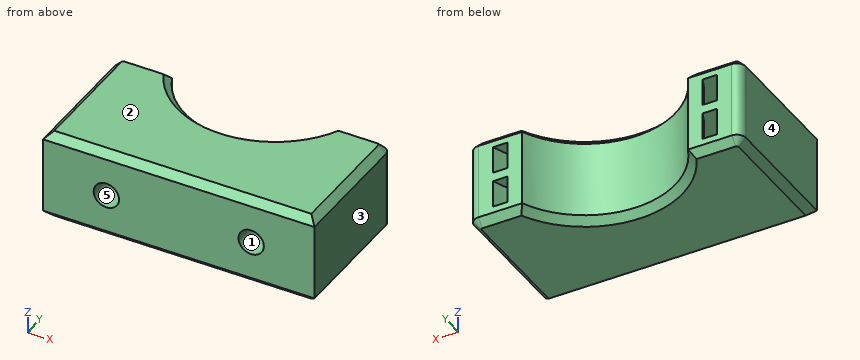
```python
from build123d import *

# Parameters (mm, degrees)
BOSS_EXTRUDE1_DEPTH = 10
SKETCH2_R           = 1.4
CUT_EXTRUDE1_DEPTH  = 6
SKETCH3_W           = 3
SKETCH3_H           = 1.5
FILLET1_R           = 1
CHAMFER1_SIZE       = 0.8


with BuildPart() as part:
    # Sketch1 → Boss-Extrude1 (new body)
    with BuildSketch(Plane.XY):
        with BuildLine():
            Line((-15, 7.5), (-15, -7.5))
            Line((-15, -7.5), (15, -7.5))
            Line((15, -7.5), (15, 7.5))
            Line((15, 7.5), (9.16515139, 7.5))
            ThreePointArc((9.16515139, 7.5), (0, 1.5), (-9.16515139, 7.5))
            Line((-9.16515139, 7.5), (-15, 7.5))
        make_face()
    extrude(amount=BOSS_EXTRUDE1_DEPTH)

    # Sketch2 → Cut-Extrude1 (cut)
    with BuildSketch(Plane.XZ.offset(7.5)):
        with Locations((-8, 5)):
            Circle(SKETCH2_R)
        with Locations((8, 5)):
            Circle(SKETCH2_R)
    extrude(amount=-CUT_EXTRUDE1_DEPTH, mode=Mode.SUBTRACT)

    # Sketch3 → Cut-Revolve1 (revolve, cut)
    with BuildSketch(Plane(origin=(0, 0, 0), x_dir=(0, 0, -1), z_dir=(1, 0, 0))):
        with Locations((-7, -0.75)):
            Rectangle(SKETCH3_W, SKETCH3_H)
        with Locations((-3, -0.75)):
            Rectangle(SKETCH3_W, SKETCH3_H)
    revolve(axis=Axis((0, 11.5, 0), (0, 0, 1)), mode=Mode.SUBTRACT)

    # Fillet1
    fillet1_edges = [part.edges().sort_by_distance(p)[0] for p in [
        (15, 7.5, 5),
        (-15, 7.5, 5),
    ]]
    fillet(fillet1_edges, radius=FILLET1_R)

    # Chamfer1
    chamfer1_edges = [part.edges().sort_by_distance(p)[0] for p in [
        (0, 1.5, 0),
        (-15, -0.5, 10),
        (0, -7.5, 10),
        (15, -0.5, 10),
        (11.582575695, 7.5, 10),
        (-11.582575695, 7.5, 0),
        (-14.707106781, 7.207106781, 0),
        (14.707106781, 7.207106781, 0),
        (-11.582575695, 7.5, 10),
        (0, 1.5, 10),
        (-14.707106781, 7.207106781, 10),
        (14.707106781, 7.207106781, 10),
        (11.582575695, 7.5, 0),
        (15, -0.5, 0),
        (0, -7.5, 0),
        (-15, -0.5, 0),
    ]]
    chamfer(chamfer1_edges, length=CHAMFER1_SIZE)


solid = part.part
```
For this review, take the finished solid that the model builds, in its own axes (mm). Face numbers are marked on the shaded views. A direction names the side the tool comes from. Coordinates: 2 decimals unless noted, no trailing zeros. Loops run counter-clockwise (first coordinate to the right, second up) from the corner with the lowest first, then second, coordinate; pieces in that order, holes last.
1. Insertion check: P1, Ø2, axis at x = -0.5, y = 2, coming from the +Z side; P2, Ø1.7, axis at x = 8, z = 5, coming from the +Y side; P3, Ø2, axis at x = 5.5, z = 8.5, coming from the +Y side. Each pin has a flat end and moves straight along its axis. Give the tip position at first contact, or say it passes through.
2. For the marked faces 4 and 5, list the 3-axis set-ups (+Z, -Z, +X, -X, +Y, -Y) from which the entire face can be reached by the end or side of a thin tool; tool diameter is ignored.
3. Mouldability with a two-part tool opening along Z and no side actions: class the marked faces 1, 2 and 3 as +Z half, -Z half, draft (parallel to the pull), parting line (faces both ways), or undercut.
4. Add section D-D, the plane y = 6. Count the separate pieces of the cut face and the enclosed holes in it, then the cut area to 3 significant figures.
5. Add section B-B, the plane y = -3. Give the boundary of the cut face in (x, z), then the cut area to 3 significant figures.
6. For line 1 (Z direction, x = -4.5, y = 0); line 2 (X direction, y = 3.75, z = 6.5); line 3 (X direction, y = 5.25, z = 8.25), list the stretches that pass through material, from the lowest coordinate up.
7. Add section C-C, the plane z = 5. Give the boundary of the cut face in (x, y).
8. Add section A-A, the plane z = 2. Give the boundary of the cut face in (x, y), then the cut area to 3 significant figures.
Result:
1. P1: stops at z = 9.71
1. P2: stops at y = 6.84
1. P3: stops at y = 3.9
2. face 4: +Z, -Z, -X, +Y, -Y
2. face 5: -Y
3. face 1: undercut
3. face 2: +Z half
3. face 3: draft
4. separate pieces: 2
4. enclosed holes: 4
4. area: 110 mm2
5. outline: (-15, 0.8) - (-14.2, 0) - (14.2, 0) - (15, 0.8) - (15, 9.2) - (14.2, 10) - (-14.2, 10) - (-15, 9.2) - close; hole circle Ø2.8 at (-8, 5); hole circle Ø2.8 at (8, 5)
5. area: 286 mm2
6. line 1: z = 0 to 1.5, 4.5 to 5.5, 8.5 to 10
6. line 2: x = -15 to -10.44, -8.5 to -6.32, 6.32 to 8.5, 10.44 to 15
6. line 3: x = -15 to -11.4, -9.65 to -7.81, 7.81 to 9.65, 11.4 to 15
7. outline: (-15, -7.5) - (-9.4, -7.5) - (-9.4, -1.5) - (-6.6, -1.5) - (-6.6, -7.5) - (6.6, -7.5) - (6.6, -1.5) - (9.4, -1.5) - (9.4, -7.5) - (15, -7.5) - (15, 6.5) arc R1 ccw to (14, 7.5) - (9.17, 7.5) arc R10 cw to (-9.17, 7.5) - (-14, 7.5) arc R1 ccw to (-15, 6.5) - close
8. outline: (-15, -7.5) - (15, -7.5) - (15, 6.5) arc R1 ccw to (14, 7.5) - (12.37, 7.5) arc R13 cw to (-12.37, 7.5) - (-14, 7.5) arc R1 ccw to (-15, 6.5) - close; (-10.78, 7.5) arc R11.5 ccw to (10.78, 7.5) - (9.17, 7.5) arc R10 cw to (-9.17, 7.5) - close
8. area: 325 mm2
